Source: CAD feature listing. Evaluate the final solid. Frame: model axes, mm. Coordinates: 2 decimals unless noted, no trailing zeros. Order: outer loops, then holes, each group sorted by start corner. A loop starts at its lowest first (then second) coordinate and runs counter-clockwise, first axis right, second up. Notation, with made-up numbers: (-27, 60) -> (13, 60) arc R30 ccw to (13, 91) -> close; hole circle Ø6 at (63, 72.25). An arc over 180 degrees is marked (long way). Put each result on its own line as item: value.
from build123d import *

# Parameters (mm, degrees)
MODEL_R             = 0.95
BOSS_EXTRUDE1_DEPTH = 1.5


with BuildPart() as part:
    # Model → Boss-Extrude1 (new body)
    with BuildSketch(Plane.XY):
        with BuildLine():
            Line((0, 108.6), (0, 5))
            ThreePointArc((0, 5), (1.464466094, 1.464466094), (5, 0))
            Line((5, 0), (365.775, 0))
            ThreePointArc((365.775, 0), (369.310533906, 1.464466094), (370.775, 5))
            Line((370.775, 5), (370.775, 108.6))
            ThreePointArc((370.775, 108.6), (369.310533906, 112.135533906), (365.775, 113.6))
            Line((365.775, 113.6), (5, 113.6))
            ThreePointArc((5, 113.6), (1.464466094, 112.135533906), (0, 108.6))
        make_face()
        with Locations((175.3875, 109.1)):
            Circle(MODEL_R, mode=Mode.SUBTRACT)
        with Locations((195.3875, 109.1)):
            Circle(MODEL_R, mode=Mode.SUBTRACT)
        Polygon((8, 8), (8, 105.6), (80.3875, 105.6), (83.3875, 109.6), (87.3875, 109.6), (90.3875, 105.6), (180.3875, 105.6), (183.3875, 109.6), (187.3875, 109.6), (190.3875, 105.6), (280.3875, 105.6), (283.3875, 109.6), (287.3875, 109.6), (290.3875, 105.6), (362.775, 105.6), (362.775, 8), (290.3875, 8), (287.3875, 4), (283.3875, 4), (280.3875, 8), (190.3875, 8), (187.3875, 4), (183.3875, 4), (180.3875, 8), (90.3875, 8), (87.3875, 4), (83.3875, 4), (80.3875, 8), align=None, mode=Mode.SUBTRACT)
        Polygon((365.947431604, 110.609548911), (367.784548911, 108.772431604), (367.112117307, 106.262882693), (364.602568396, 105.590451089), (362.765451089, 107.427568396), (363.437882693, 109.937117307), align=None, mode=Mode.SUBTRACT)
        Polygon((4.827568396, 110.609548911), (2.990451089, 108.772431604), (3.662882693, 106.262882693), (6.172431604, 105.590451089), (8.009548911, 107.427568396), (7.337117307, 109.937117307), align=None, mode=Mode.SUBTRACT)
        Polygon((365.947431604, 2.990451089), (367.784548911, 4.827568396), (367.112117307, 7.337117307), (364.602568396, 8.009548911), (362.765451089, 6.172431604), (363.437882693, 3.662882693), align=None, mode=Mode.SUBTRACT)
        Polygon((126.799038106, 2.25), (124.200961894, 2.25), (122.901923789, 4.5), (124.200961894, 6.75), (126.799038106, 6.75), (128.098076211, 4.5), align=None, mode=Mode.SUBTRACT)
        Polygon((4.827568396, 2.990451089), (2.990451089, 4.827568396), (3.662882693, 7.337117307), (6.172431604, 8.009548911), (8.009548911, 6.172431604), (7.337117307, 3.662882693), align=None, mode=Mode.SUBTRACT)
        Polygon((243.975961894, 2.25), (246.574038106, 2.25), (247.873076211, 4.5), (246.574038106, 6.75), (243.975961894, 6.75), (242.676923789, 4.5), align=None, mode=Mode.SUBTRACT)
        Polygon((126.799038106, 111.35), (124.200961894, 111.35), (122.901923789, 109.1), (124.200961894, 106.85), (126.799038106, 106.85), (128.098076211, 109.1), align=None, mode=Mode.SUBTRACT)
        Polygon((243.975961894, 111.35), (246.574038106, 111.35), (247.873076211, 109.1), (246.574038106, 106.85), (243.975961894, 106.85), (242.676923789, 109.1), align=None, mode=Mode.SUBTRACT)
    extrude(amount=BOSS_EXTRUDE1_DEPTH)


solid = part.part
1. Cut plane B-B on x = 40. Output: boundary loops of the cut face in (y, z).
Numbers:
outline: (0, 0) -> (8, 0) -> (8, 1.5) -> (0, 1.5) -> close; (105.6, 0) -> (113.6, 0) -> (113.6, 1.5) -> (105.6, 1.5) -> close
2. Cut plane A-A on y = 68.5. Output: boundary loops of the cut face in (x, z) (3 decimals).
Numbers:
outline: (0, 0) -> (8, 0) -> (8, 1.5) -> (0, 1.5) -> close; (362.775, 0) -> (370.775, 0) -> (370.775, 1.5) -> (362.775, 1.5) -> close
3. Cut plane C-C on z = 0.6. Count the separate pieces of the cut face and the enclosed holes in it, plus the area to 3 significant figures.
Numbers:
separate pieces: 1
enclosed holes: 11
area: 7,160 mm2
4. Ray query, line 1 along Y through (x, z) = (217, 0.9); line 2 along X through (y, z) = (42, 0.45) (3 decimals); line 3 along Y through (x, z) = (195.5, 1.05). Return the intervals inside material, ascending.
Numbers:
line 1: y = 0 to 8, 105.6 to 113.6
line 2: x = 0 to 8, 362.775 to 370.775
line 3: y = 0 to 8, 105.6 to 108.16, 110.04 to 113.6
